Geometry check sheet. Reference: the model listing, model coordinates, mm. A direction names the side the tool comes from. Round coordinates to 2 decimals unless told otherwise and drop trailing zeros. Write each loop counter-clockwise with the first axis right and the second up, starting at its lowest first coordinate (ties: lowest second). Pieces come first, ordered by that corner, then holes.
Item 1: Draft check along Z on faces 3 (the face through (0, -35, 5.3)), 4 (the face through (1.588, -32.105, 6.187)), 5 (the face through (2, -35, 7.1)). Enter one of: pulls with the +Z half, pulls with the -Z half, needs draft (parallel to the pull), parting line crosses it, or undercut.
Item 2: Cross-section at D-D (z = 7.8). Enter the section's corners in (x, y) (3 decimals), then the cut area to 3 significant figures.
Item 3: Cross-section at B-B (x = 2.2). Enter the section's corners in (y, z).
Item 4: Depth check by flat-ended pin: P1, Ø1.5, axis at x = 0.5, z = 9, coming from the +Y side (3 decimals); P2, Ø1.5, axis at y = -32.5, z = 7, coming from the +X side; P3, Ø1.5, axis at x = 1, z = 6.5, coming from the +Y side. Enter the tip coordinate at first touch or a pass-through.
Item 5: Cross-section at A-A (z = 6.6). Enter the section's corners in (x, y) (3 decimals).
Item 6: Scan lines: probe 1 along Z at (x, y) = (1.5, -36.05); probe 2 along Y at (x, z) = (0.05, 7.2); probe 3 along Y at (x, z) = (0.6, 7.15). Record each from-to range of solid material in increasing order.
Item 7: Cross-section at C-C (y = -32.05). Enter the section's corners in (x, z), then the cut area to 3 significant figures.
Item 8: Access from +Z, -Z, +X, -X, +Y, -Y to the whole of each face (thin tool, end or side, straight path). Record for faces 1 (the face through (0, -35, 9.5)), 2 (the face through (-0.44, -36.49, 7.91)).
from build123d import *

# Parameters (mm, degrees)
CYLINDER007_R     = 1.9
CYLINDER007_DEPTH = 2.4
CYLINDER006_R     = 3
CYLINDER006_DEPTH = 1.8
FILLET004_R       = 0.75


with BuildPart() as cylinder011:
    # Cylinder007 → Cylinder007 (new body)
    with BuildSketch(Plane.XY.offset(1.5)):
        Circle(CYLINDER007_R)
    extrude(amount=CYLINDER007_DEPTH)


with BuildPart() as obj1:
    # Cylinder006 → Cylinder006 (new body)
    with BuildSketch(Plane.XY.offset(-0.3)):
        Circle(CYLINDER006_R)
    extrude(amount=CYLINDER006_DEPTH)

    # Fusion017: union Cylinder011
    add(cylinder011.part)

    # Fillet004
    fillet004_edges = [obj1.edges().sort_by_distance(p)[0] for p in [
        (-1.9, 0, 3.9),
    ]]
    fillet(fillet004_edges, radius=FILLET004_R)


with BuildPart() as obj1_1:
    # Fillet004 placement: moved
    add(obj1.part.moved(Location((-0.025, -34.635, 5.6))))


solid = obj1_1.part
Resolved:
1. face 3: pulls with the -Z half
1. face 4: needs draft
1. face 5: pulls with the +Z half
2. outline: circle Ø3.8 at (-0.025, -34.635)
2. area: 11.3 mm2
3. outline: (-36.65, 5.3) - (-32.62, 5.3) - (-32.62, 7.1) - (-36.65, 7.1) - close
4. P1: stops at y = -32.735
4. P2: stops at x = 2.64
4. P3: stops at y = -31.65
5. outline: circle Ø6 at (-0.025, -34.635)
6. probe 1: z = 5.3 to 7.1
6. probe 2: y = -36.53 to -32.74
6. probe 3: y = -36.43 to -32.84
7. outline: (-1.55, 5.3) - (1.5, 5.3) - (1.5, 7.1) - (-1.55, 7.1) - close
7. area: 5.48 mm2
8. face 1: +Z, +X, -X, +Y, -Y
8. face 2: +Z
